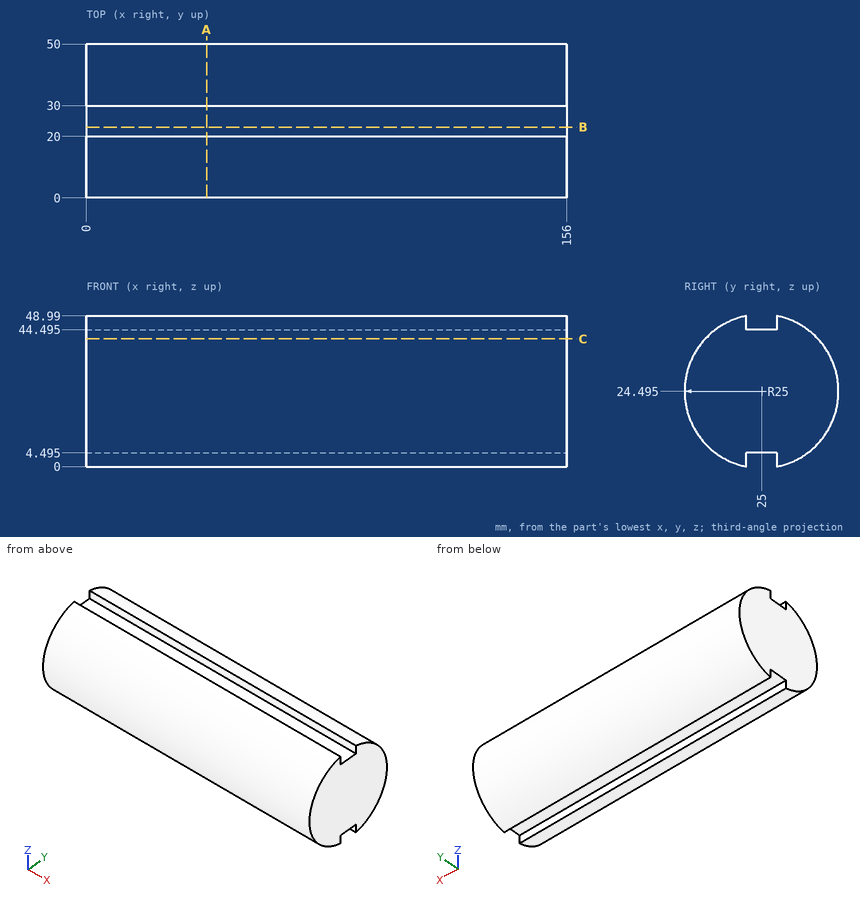
For this review, use the dimensioned drawing (mm, ordinates from the lowest corner) and the shaded views. Coordinates: 2 decimals unless noted, no trailing zeros. Loops run counter-clockwise (first coordinate to the right, second up) from the corner with the lowest first, then second, coordinate; pieces in that order, holes last. Notation, with made-up numbers: (17, -26) -> (26, -26) arc R32 cw to (26, 8) -> close; hole circle Ø9 at (70.25, -31.5). An arc over 180 degrees is marked (long way). Use a Markdown table: item, result. Add a question column.
1. Add section A-A on x = 39. Write out the cut boundary in (y, z) (1 decimal).
2. Add section B-B on y = 23. Write out the cut boundary in (x, z) (1 decimal), plus the area to 3 significant figures.
3. Clearance check with flat-ended pins moving along their axes: pin 1 Ø12 at (x, y) = (64.5, 16.5) entering from -Z; pin 2 Ø6 at (x, z) = (112.5, 33) entering from +Y; pin 3 Ø5 at (x, y) = (111, 45) entering from +Z. State where each tip first meets the part, or that it passes through.
4. To check wall thickness, follow line 1 (Z direction, x = 47, y = 23) (1 decimal); line 2 (Y direction, x = 12.5, z = 47) (1 decimal); line 3 (Y direction, x = 134, z = 46). State the ranges of each line that lie inside material, in increasing order.
5. Add section C-C on z = 41.5. Write out the cut boundary in (x, y).
Returned:
| question | item | result |
|---|---|---|
| 1 | outline | (20, 0) -> (20, 4.5) -> (30, 4.5) -> (30, 0) arc R25 ccw to (30, 49) -> (30, 44.5) -> (20, 44.5) -> (20, 49) arc R25 ccw to start |
| 2 | outline | (0, 4.5) -> (156, 4.5) -> (156, 44.5) -> (0, 44.5) -> close |
| 2 | area | 6,240 mm² |
| 3 | pin 1 | stops at z = 0 |
| 3 | pin 2 | stops at y = 49.39 |
| 3 | pin 3 | stops at z = 42.35 |
| 4 | line 1 | z = 4.5 to 44.5 |
| 4 | line 2 | y = 14.1 to 20, 30 to 35.9 |
| 4 | line 3 | y = 12.25 to 20, 30 to 37.75 |
| 5 | outline | (0, 6.67) -> (156, 6.67) -> (156, 43.33) -> (0, 43.33) -> close |
